The listing builds one solid part. Answer for the finished solid, in the listing's coordinates (mm). Give positions to 0.01 mm unless a question says otherwise; leave off trailing zeros. Order: outer loops, then holes, each group sorted by start corner. A loop starts at its lowest first (then second) coordinate and runs counter-clockwise, first axis right, second up. Notation, with made-up numbers: (66.5, 11.5) - (82.5, 11.5) arc R24 ccw to (82.5, 37.5) - close; hole circle Ø1 at (-21.75, 31.5). An arc over 180 degrees is marked (long way). Use a Markdown table: item, result. Add a question column.
1) Straight lines are drawn through the part: line 1 (Z direction, x = 0, y = 1.9); line 2 (X direction, y = 1.9, z = 0). For each, find the intervals that lie inside material, in ascending order.
2) Find section D-D, the plane x = -1.5. Determine the outline of the cut face in (y, z), plus the area to 3 significant figures.
3) Find section A-A, the plane y = 0.95. Determine the outline of the cut face in (x, z).
4) Find section C-C, the plane x = 0. Determine the outline of the cut face in (y, z), plus the area to 3 significant figures.
5) Find section B-B, the plane z = 0. Determine the outline of the cut face in (x, y).
6) A flat-ended cylindrical pin translates along its axis: pin 1 (1.8 mm diameter, centred on x = -1.5, z = 0, fed in from -Y). Find the tip coordinate at first contact, or state that the pin passes through.
from build123d import *

# Parameters (mm, degrees)
EXTRUDE_THIN3_DEPTH     = 3.1
SKETCH2_W               = 2.4
SKETCH2_H               = 1
CUT_EXTRUDE1_DEPTH      = 4.1
CUT_EXTRUDE1_DEPTH_BACK = 4.1
SKETCH3_W               = 2.4
SKETCH3_H               = 0.15
CUT_EXTRUDE2_DEPTH      = 1
FILLET1_R               = 0.15
SKETCH4_R               = 1.6
CUT_EXTRUDE3_DEPTH      = 1


with BuildPart() as part:
    # Sketch1 → Extrude-Thin3 (new body, symmetric)
    with BuildSketch(Plane(origin=(0, 0, 0), x_dir=(0, 0, -1), z_dir=(1, 0, 0))):
        Polygon((-3.1, 0.2), (-3.1, 2), (3.1, 2), (3.1, 0.2), (2.95, 0.2), (2.95, 1.85), (-2.95, 1.85), (-2.95, 0.2), align=None)
    extrude(amount=EXTRUDE_THIN3_DEPTH, both=True)

    # Sketch2 → Cut-Extrude1 (cut, two sides)
    with BuildSketch(Plane.XY) as cut_extrude1_sk:
        with Locations((0, 1.35)):
            Rectangle(SKETCH2_W, SKETCH2_H)
        Polygon((-3.1, 1.3), (-2, 0.2), (-3.1, 0.2), align=None)
        Polygon((3.1, 0.2), (3.1, 1.3), (2, 0.2), align=None)
    extrude(amount=CUT_EXTRUDE1_DEPTH, mode=Mode.SUBTRACT)
    extrude(cut_extrude1_sk.sketch, amount=-CUT_EXTRUDE1_DEPTH_BACK, mode=Mode.SUBTRACT)

    # Sketch3 → Cut-Extrude2 (cut)
    with BuildSketch(Plane(origin=(0, 2, 0), x_dir=(1, 0, 0), z_dir=(0, 1, 0))):
        with Locations((0, 3.025)):
            Rectangle(SKETCH3_W, SKETCH3_H)
        with Locations((0, -3.025)):
            Rectangle(SKETCH3_W, SKETCH3_H)
    extrude(amount=-CUT_EXTRUDE2_DEPTH, mode=Mode.SUBTRACT)

    # Fillet1
    fillet1_edges = [part.edges().sort_by_distance(p)[0] for p in [
        (-2.15, 2, -3.1),
        (2.15, 2, -3.1),
        (-2.15, 2, 3.1),
        (2.15, 2, 3.1),
    ]]
    fillet(fillet1_edges, radius=FILLET1_R)

    # Sketch4 → Cut-Extrude3 (cut)
    with BuildSketch(Plane(origin=(0, 2, 0), x_dir=(1, 0, 0), z_dir=(0, 1, 0))):
        Circle(SKETCH4_R)
    extrude(amount=-CUT_EXTRUDE3_DEPTH, mode=Mode.SUBTRACT)


solid = part.part
The answers:
| question | item | result |
|---|---|---|
| 1 | line 1 | -2.95 to -1.6, 1.6 to 2.95 |
| 1 | line 2 | -3.1 to -1.6, 1.6 to 3.1 |
| 2 | outline | (0.2, -3.1) - (1.85, -3.1) arc R0.15 ccw to (2, -2.95) - (2, -0.56) - (1.85, -0.56) - (1.85, -2.95) - (0.2, -2.95) - close; (0.2, 2.95) - (1.85, 2.95) - (1.85, 0.56) - (2, 0.56) - (2, 2.95) arc R0.15 ccw to (1.85, 3.1) - (0.2, 3.1) - close |
| 2 | area | 1.25 mm2 |
| 3 | outline | (-2.75, -3.1) - (-1.2, -3.1) - (-1.2, -2.95) - (-2.75, -2.95) - close; (-2.75, 2.95) - (-1.2, 2.95) - (-1.2, 3.1) - (-2.75, 3.1) - close; (1.2, -3.1) - (2.75, -3.1) - (2.75, -2.95) - (1.2, -2.95) - close; (1.2, 2.95) - (2.75, 2.95) - (2.75, 3.1) - (1.2, 3.1) - close |
| 4 | outline | (0.2, -3.1) - (0.85, -3.1) - (0.85, -2.95) - (0.2, -2.95) - close; (0.2, 2.95) - (0.85, 2.95) - (0.85, 3.1) - (0.2, 3.1) - close; (1.85, -2.95) - (2, -2.95) - (2, -1.6) - (1.85, -1.6) - close; (1.85, 1.6) - (2, 1.6) - (2, 2.95) - (1.85, 2.95) - close |
| 4 | area | 0.600 mm2 |
| 5 | outline | (-3.1, 1.85) - (-1.6, 1.85) - (-1.6, 2) - (-3.1, 2) - close; (1.6, 1.85) - (3.1, 1.85) - (3.1, 2) - (1.6, 2) - close |
| 6 | pin 1 | y = 1.85 |
